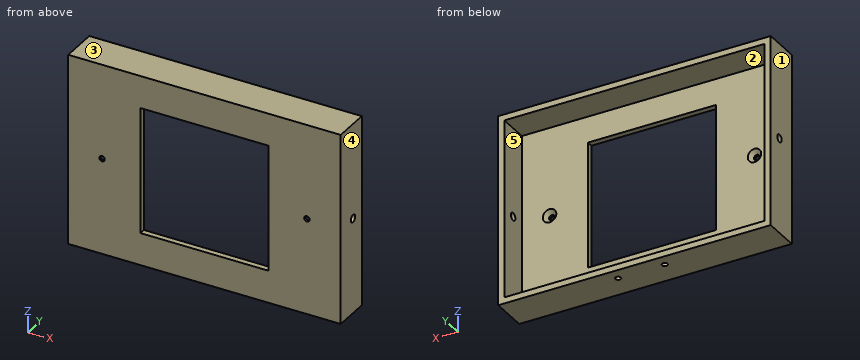
```python
from build123d import *

# Parameters (mm, degrees)
SKETCH1_W                                       = 89.09
SKETCH1_H                                       = 62.42
SKETCH1_W_2                                     = 85.09
SKETCH1_H_2                                     = 58.42
BOSS_EXTRUDE1_DEPTH                             = 2
SKETCH1_3_W                                     = 89.09
SKETCH1_3_H                                     = 62.42
SKETCH1_3_W_2                                   = 85.09
SKETCH1_3_H_2                                   = 58.42
BOSS_EXTRUDE2_DEPTH                             = 10
CSK_FOR_M2_FLAT_HEAD_MACHINE_SCREW1_D           = 1.8
CSK_FOR_M2_FLAT_HEAD_MACHINE_SCREW1_DEPTH       = 9.906
CSK_FOR_M2_FLAT_HEAD_MACHINE_SCREW1_CSINK_D     = 4.4
CSK_FOR_M2_FLAT_HEAD_MACHINE_SCREW1_CSINK_ANGLE = 90
CSK_FOR_M2_FLAT_HEAD_MACHINE_SCREW1_TIP         = 0.540774557
SKETCH7_W                                       = 41.935160688
SKETCH7_H                                       = 41.279429724
CUT_EXTRUDE1_DEPTH                              = 2.54
CUT_EXTRUDE2_REACH                              = 79.334
SKETCH8_R                                       = 0.9
SKETCH9_R                                       = 1.25
CUT_EXTRUDE3_DEPTH                              = 95.92677283


with BuildPart() as part:
    # Sketch1 → Boss-Extrude1 (new body)
    # profile 1 of 2: a face of its own
    with BuildSketch(Plane(origin=(0, 0, 0), x_dir=(1, 0, 0), z_dir=(0, 1, 0))):
        Rectangle(SKETCH1_W, SKETCH1_H)
        Rectangle(SKETCH1_W_2, SKETCH1_H_2, mode=Mode.SUBTRACT)
    # profile 2 of 2: a face of its own
    with BuildSketch(Plane(origin=(0, 0, 0), x_dir=(1, 0, 0), z_dir=(0, 1, 0))):
        Rectangle(SKETCH1_W_2, SKETCH1_H_2)
    extrude(amount=-BOSS_EXTRUDE1_DEPTH)

    # Sketch1_3 → Boss-Extrude2 (add)
    with BuildSketch(Plane(origin=(0, 0, 0), x_dir=(1, 0, 0), z_dir=(0, 1, 0))):
        Rectangle(SKETCH1_3_W, SKETCH1_3_H)
        Rectangle(SKETCH1_3_W_2, SKETCH1_3_H_2, mode=Mode.SUBTRACT)
    extrude(amount=BOSS_EXTRUDE2_DEPTH)

    # CSK for M2 Flat Head Machine Screw1
    with Locations(Plane(origin=(0, 0, 0), x_dir=(1, 0, 0), z_dir=(0, 1, 0))):
        with Locations((-33.5, -0.21892606), (33.5, -0.21892606)):
            CounterSinkHole(CSK_FOR_M2_FLAT_HEAD_MACHINE_SCREW1_D / 2, CSK_FOR_M2_FLAT_HEAD_MACHINE_SCREW1_CSINK_D / 2, depth=CSK_FOR_M2_FLAT_HEAD_MACHINE_SCREW1_DEPTH, counter_sink_angle=CSK_FOR_M2_FLAT_HEAD_MACHINE_SCREW1_CSINK_ANGLE)
            with Locations((0, 0, -(CSK_FOR_M2_FLAT_HEAD_MACHINE_SCREW1_DEPTH + CSK_FOR_M2_FLAT_HEAD_MACHINE_SCREW1_TIP / 2))):  # 118° drill point
                Cone(0, CSK_FOR_M2_FLAT_HEAD_MACHINE_SCREW1_D / 2, CSK_FOR_M2_FLAT_HEAD_MACHINE_SCREW1_TIP, mode=Mode.SUBTRACT)

    # Sketch7 → Cut-Extrude1 (cut)
    with BuildSketch(Plane(origin=(0, 0, 0), x_dir=(1, 0, 0), z_dir=(0, 1, 0))):
        Rectangle(SKETCH7_W, SKETCH7_H)
    extrude(amount=-CUT_EXTRUDE1_DEPTH, mode=Mode.SUBTRACT)

    # Sketch8 → Cut-Extrude2 (cut, up to next)
    with BuildSketch(Plane(origin=(0, 0, -31.21), x_dir=(-1, 0, 0), z_dir=(0, 0, -1)), mode=Mode.PRIVATE) as cut_extrude2_sk1:
        with Locations((-7.635, 6)):
            Circle(SKETCH8_R)
    cut_extrude2_tool1 = extrude(cut_extrude2_sk1.sketch, amount=-CUT_EXTRUDE2_REACH, mode=Mode.PRIVATE) & part.part
    # Sketch8 → Cut-Extrude2 (cut, up to next)
    with BuildSketch(Plane(origin=(0, 0, -31.21), x_dir=(-1, 0, 0), z_dir=(0, 0, -1)), mode=Mode.PRIVATE) as cut_extrude2_sk2:
        with Locations((7.635, 6)):
            Circle(SKETCH8_R)
    cut_extrude2_tool2 = extrude(cut_extrude2_sk2.sketch, amount=-CUT_EXTRUDE2_REACH, mode=Mode.PRIVATE) & part.part
    add(cut_extrude2_tool1.solids().sort_by_distance((7.635, 6, -31.21))[0], mode=Mode.SUBTRACT)
    add(cut_extrude2_tool2.solids().sort_by_distance((-7.635, 6, -31.21))[0], mode=Mode.SUBTRACT)

    # Sketch9 → Cut-Extrude3 (cut, through all)
    with BuildSketch(Plane(origin=(44.545, 0, 0), x_dir=(0, 0, -1), z_dir=(1, 0, 0))):
        with Locations((0, 5)):
            Circle(SKETCH9_R)
    extrude(amount=-CUT_EXTRUDE3_DEPTH, mode=Mode.SUBTRACT)


solid = part.part
```
Input: part model. Units: mm. Frame: model coordinates. Face numbers are marked on the shaded views. A direction names the side the tool comes from. Round coordinates to 2 decimals unless told otherwise and drop trailing zeros. Loops run counter-clockwise (first coordinate to the right, second up) from the corner with the lowest first, then second, coordinate; pieces in that order, holes last. Notation, with made-up numbers: (66, 84) -> (109, 84) arc R13 ccw to (109, 88) -> close; hole circle Ø6 at (28.5, -12.75). An arc over 180 degrees is marked (long way). Use one line per item in the form item = value. Start each with the question number.
Item 1: Mould query, pull axis X, two halves, no side actions, for the marked faces 3, 4 and 5. Classes: pulls with the +X half, pulls with the -X half, needs draft (parallel to the pull), parting line crosses it, or undercut.
Item 2: Material intervals for L1, parallel to Y at x = -43, z = 0; L2, parallel to X at y = 2.5, z = 0.5 (3 decimals); L3, parallel to Z at x = -9.5, y = 4.75, sorted ascending. Write a range as from..to.
Item 3: Section query B-B on z = 5.5. Return the cut outline in (x, y) (3 decimals).
Item 4: Contact query for flat-ended pins moving along their axis: pin 1 Ø2 at (y, z) = (5, 0) entering from +X; pin 2 Ø10 at (x, z) = (-30, -3.5) entering from +Y. Output: stop coordinate, or through.
Item 5: Section query C-C on x = 2.5. Return the cut outline in (y, z), then the cut area to 3 significant figures.
Item 6: Section query D-D on z = -24. Return the cut outline in (x, y) (3 decimals), then the cut area to 3 significant figures.
Item 7: Set-up query: the marked faces 1 and 2. Return all of +Z, -Z, +X, -X, +Y, -Y with unobstructed straight access to the full face (end or side cutting, diameter ignored); none if empty.
Item 8: Section query A-A on x = 33.5. Return the cut outline in (y, z).
Ans:
q1.face_3 = needs draft
q1.face_4 = pulls with the +X half
q1.face_5 = undercut
q2.L1 = -2..3.75, 6.25..10
q2.L2 = -44.545..-42.545, 42.545..44.545
q2.L3 = -31.21..-29.21, 29.21..31.21
q3.outline = (-44.545, -2) -> (-20.968, -2) -> (-20.968, 0) -> (-42.545, 0) -> (-42.545, 10) -> (-44.545, 10) -> close; (20.968, -2) -> (44.545, -2) -> (44.545, 10) -> (42.545, 10) -> (42.545, 0) -> (20.968, 0) -> close
q4.pin_1 = through
q4.pin_2 = 0
q5.outline = (-2, -31.21) -> (10, -31.21) -> (10, -29.21) -> (0, -29.21) -> (0, -20.64) -> (-2, -20.64) -> close; (-2, 20.64) -> (0, 20.64) -> (0, 29.21) -> (10, 29.21) -> (10, 31.21) -> (-2, 31.21) -> close
q5.area = 82.3 mm^2
q6.outline = (-44.545, -2) -> (44.545, -2) -> (44.545, 10) -> (42.545, 10) -> (42.545, 0) -> (-42.545, 0) -> (-42.545, 10) -> (-44.545, 10) -> close
q6.area = 218 mm^2
q7.face_1 = +Z, -Z, -X, +Y, -Y
q7.face_2 = +Y
q8.outline = (-2, -31.21) -> (10, -31.21) -> (10, -29.21) -> (0, -29.21) -> (0, -1.98) -> (-1.3, -0.68) -> (-2, -0.68) -> close; (-2, 1.12) -> (-1.3, 1.12) -> (0, 2.42) -> (0, 29.21) -> (10, 29.21) -> (10, 31.21) -> (-2, 31.21) -> close
